Input: part model. Units: mm. Frame: model coordinates. A direction names the side the tool comes from. Coordinates: 2 decimals unless noted, no trailing zeros. Use a Markdown table: item, result. Add a question column.
1. Pin query (flat end, axial travel): pin 1 (4 mm diameter, centred on x = -12, z = -35, fed in from +Y); pin 2 (10 mm diameter, centred on x = 4, z = -36.5, fed in from -Y); pin 3 (4 mm diameter, centred on x = 7.5, y = -8.5, fed in from -Z). Return the tip coordinate at first contact, or that it passes through.
2. Line query: L1, parallel to Y at x = -6.5, z = -30; L2, parallel to Y at x = -6, z = 5; L3, parallel to Z at x = 18.5, y = 7.5. Output: solid intervals per line, ascending. Write a range as [from, to].
3. Set-up query: faces 5 (the cylindrical face through (-15.28, -3.41, 11.43)), 6 (the cylindrical face through (14.684, -2.082, -0.601)). Return all of +Z, -Z, +X, -X, +Y, -Y with unobstructed straight access to the full face (end or side cutting, diameter ignored); none if empty.
4. Draft query along Y for faces 1 (the cylindrical face through (-18.03, 30.4, 5.64)), 2 (the cylindrical face through (-14.751, 40.047, -32.696)), 3 (the cylindrical face through (17.437, 34.453, 2.954)), 4 (the cylindrical face through (26.653, -28.781, 3.168)). Return one class per face: +Y half, -Y half, draft (parallel to the pull), parting line (faces both ways), or undercut.
```python
from build123d import *

# Parameters (mm, degrees)
RESSALTO_EXTRUS_O1_DEPTH   = 12
RESSALTO_EXTRUS_O2_DEPTH   = 12
RESSALTO_EXTRUS_O3_DEPTH   = 12
FILETE1_R                  = 10
FILETE2_R                  = 2
FILETE3_R                  = 2
ESBO_O11_R                 = 3.1
CORTE_EXTRUS_O4_DEPTH      = 40
ESBO_O12_R                 = 3.1
CORTE_EXTRUS_O5_DEPTH      = 40
ESBO_O10_R                 = 3.1
CORTE_EXTRUS_O6_DEPTH      = 40
CORTE_EXTRUS_O8_DEPTH      = 10
CORTE_EXTRUS_O8_DEPTH_BACK = 30
ESBO_O15_R                 = 3


with BuildPart() as part:
    # Esboço1 → Ressalto-extrusão1 (new body)
    with BuildSketch(Plane.XY):
        Polygon((7.254630019, -29.35114002), (-37.745369981, 20.64885998), (-37.745369981, 40.64885998), (27.254630019, 40.64885998), (27.254630019, -29.35114002), align=None)
    extrude(amount=RESSALTO_EXTRUS_O1_DEPTH)

    # Esboço2 → Ressalto-extrusão2 (add)
    with BuildSketch(Plane(origin=(0, 40.64885998, 0), x_dir=(1, 0, 0), z_dir=(0, 1, 0))):
        Polygon((7.254630019, 58), (-37.745369981, 8), (-37.745369981, -12), (27.254630019, -12), (27.254630019, 58), align=None)
    extrude(amount=-RESSALTO_EXTRUS_O2_DEPTH)

    # Esboço3 → Ressalto-extrusão3 (add)
    with BuildSketch(Plane(origin=(27.254630019, 0, 0), x_dir=(0, 0, -1), z_dir=(1, 0, 0))):
        Polygon((58, 20.64885998), (8, -29.35114002), (-12, -29.35114002), (-12, 40.64885998), (58, 40.64885998), align=None)
    extrude(amount=-RESSALTO_EXTRUS_O3_DEPTH)

    # Filete1
    filete1_edges = [part.edges().sort_by_distance(p)[0] for p in [
        (-37.745369981, 34.64885998, -8),
        (7.254630019, 34.64885998, -58),
        (21.254630019, -29.35114002, -8),
        (21.254630019, 20.64885998, -58),
        (7.254630019, -29.35114002, 6),
        (-37.745369981, 20.64885998, 6),
    ]]
    fillet(filete1_edges, radius=FILETE1_R)

    # Filete2
    filete2_edges = [part.edges().sort_by_distance(p)[0] for p in [
        (-37.745369981, 32.567540006, 12),
        (19.481442042, 40.64885998, -58),
        (27.254630019, 5.64885998, 12),
        (-15.45149942, 40.64885998, -32.77096729),
        (7.639868216, 40.64885998, -57.135000634),
        (-37.081574098, 40.64885998, -7.74527762),
        (-15.45149942, -4.12210731, 12),
        (19.481442042, -29.35114002, 12),
        (7.639868216, -28.486140654, 12),
        (-37.081574098, 20.90358236, 12),
        (27.254630019, -4.35114002, -33),
        (27.254630019, 32.719927792, -58),
        (27.254630019, 20.96416128, -57.238795325),
        (27.254630019, -28.589935345, -7.6846987),
        (-5.245369981, 40.64885998, 12),
        (27.254630019, -29.35114002, 4.071067812),
        (-37.745369981, 40.64885998, 3.918680026),
        (27.254630019, 40.64885998, -23),
    ]]
    fillet(filete2_edges, radius=FILETE2_R)

    # Filete3
    filete3_edges = [part.edges().sort_by_distance(p)[0] for p in [
        (-11.245369981, 28.64885998, 0),
        (15.254630019, -0.35114002, 0),
        (15.254630019, 28.64885998, -29),
    ]]
    fillet(filete3_edges, radius=FILETE3_R)

    # Esboço11 → Corte-extrusão4 (cut)
    with BuildSketch(Plane.ZY.offset(37.745369981)):
        with Locations(Location((4.707106781, 33.355966761, 0), (0, 0, 270))):
            Circle(ESBO_O11_R)
    extrude(amount=-CORTE_EXTRUS_O4_DEPTH, mode=Mode.SUBTRACT)

    # Esboço12 → Corte-extrusão5 (cut)
    with BuildSketch(Plane.XZ.offset(29.35114002)):
        with Locations(Location((19.9617368, 4.707106781, 0), (0, 0, 270))):
            Circle(ESBO_O12_R)
    extrude(amount=-CORTE_EXTRUS_O5_DEPTH, mode=Mode.SUBTRACT)

    # Esboço10 → Corte-extrusão6 (cut)
    with BuildSketch(Plane(origin=(0, 0, -58), x_dir=(-1, 0, 0), z_dir=(0, 0, -1))):
        with Locations((-19.9617368, 33.355966761)):
            Circle(ESBO_O10_R)
    extrude(amount=-CORTE_EXTRUS_O6_DEPTH, mode=Mode.SUBTRACT)

    # Esboço15 → Corte-extrusão8 (cut, two sides: drawn at the far end of the back side and taken through both)
    with BuildSketch(Plane(origin=(25.301163333, 25.301163333, 25.301163333), x_dir=(0.8164965809277263, -0.40824829046386346, -0.40824829046386246), z_dir=(0.5773502691896256, 0.5773502691896265, 0.5773502691896252)).offset(-CORTE_EXTRUS_O8_DEPTH_BACK)):
        with Locations(Location((1.188623136, 20.258589603, 0), (0, 0, 320.328232449))):
            Circle(ESBO_O15_R)
    extrude(amount=CORTE_EXTRUS_O8_DEPTH + CORTE_EXTRUS_O8_DEPTH_BACK, mode=Mode.SUBTRACT)


solid = part.part
```
Answers below:
| question | item | result |
|---|---|---|
| 1 | pin 1 | stops at y = 40.65 |
| 1 | pin 2 | stops at y = 28.65 |
| 1 | pin 3 | stops at z = 0 |
| 2 | L1 | y = [28.65, 40.65] |
| 2 | L2 | y = [-14.62, 30.27], [36.44, 40.65] |
| 2 | L3 | z = [-44.85, 1.97], [7.44, 12] |
| 3 | face 5 | +Z, -X, -Y |
| 3 | face 6 | -Z, -X, -Y |
| 4 | face 1 | undercut |
| 4 | face 2 | +Y half |
| 4 | face 3 | undercut |
| 4 | face 4 | -Y half |
